Geometry: final body of the model. Coordinates: model frame, mm. Face numbers are marked on the shaded views. A direction names the side the tool comes from. Give positions to 0.01 mm unless a question says otherwise; leave off trailing zeros. One line per item, written item: value. Start each with the question number.
Autodesk Inventor part; units mm, degrees
ref_plane "YZ Plane" through (0, 0, 0) normal (1, 0, 0) x (0, 1, 0)
ref_plane "XZ Plane" through (0, 0, 0) normal (0, 1, 0) x (-1, 0, 0)
ref_plane "XY Plane" through (0, 0, 0) normal (0, 0, 1) x (1, 0, 0)
sketch "Sketch1" plane through (0, 0, 0) normal (0, 0, 1) x (1, 0, 0)
  line L0 (0, 0) -> (0, 190.5)
  line L1 (0, 190.5) -> (1.524, 190.5)
  line L2 (1.524, 190.5) -> (1.524, 260.35)
  line L3 (1.524, 260.35) -> (50.8, 260.35)
  line L4 (50.8, 260.35) -> (50.8, 187.325)
  line L5 (50.8, 187.325) -> (115.7676, 161.925)
  line L6 (115.7676, 161.925) -> (130.048, 161.925)
  line L7 (130.048, 161.925) -> (130.048, 0)
  line L8 (130.048, 0) -> (0, 0)
  line L9 (130.048, 160.3375) -> (0, 160.3375)
  dimension "d0" = 520.7
  dimension "d1" = 381
  dimension "d2" = 1.524
  dimension "d3" = 320.675
  dimension "d4" = 323.85
  dimension "d7" = 374.65
  dimension "d18" = 49.276
  dimension "d20" = 128.524
  dimension "d21" = 14.2804
revolve "Revolution1" add sketch "Sketch1" angle 360 about axis through (130.048, 0, 0) along (-1, 0, 0) contours L0 L1 L2 L3 L4 L5 L6 L7 L9
sketch "Sketch2" plane through (1.524, 0, 0) normal (-1, 0, 0) x (0, 0, 1)
  circle A0 centre (0, 0) radius 260.35
  circle A1 centre (0, 0) radius 190.5
  circle A2 centre (221.0935, 43.9782) radius 15.875
  line L0 (221.0935, 43.9782) -> (0, 0) construction
  circle A3 centre (0, 0) radius 225.425 construction
  line L1 (0, 0) -> (225.425, 0) construction
  dimension "d10" = 225.425
  dimension "d11" = 31.75
  dimension "d17" = 11.25
extrude "Extrusion1" cut sketch "Sketch2" against normal through all contours A2
pattern_circular "Circular Pattern1" count 16 over 360 about axis through (83.2838, 0, 0) along (1, 0, 0) of "Extrusion1"
chamfer "Chamfer1" distance 1.5875 angle 45 2 edges at (1.524, -260.35, 0) (50.8, -260.35, 0)
sketch "Sketch3" plane through (0, 0, 0) normal (0, 1, 0) x (-1, 0, 0)
  line L0 (-50.8, 187.325) -> (-115.7676, 161.925) construction
  line L1 (-115.7676, 161.925) -> (-130.048, 161.925) construction
  line L2 (-130.048, 160.3375) -> (0, 160.3375) construction
  line L3 (26.0096, 0) -> (-156.0576, 0)
  line L4 (-25.4, 160.3375) -> (-130.048, 160.3375)
  line L5 (-130.048, 160.3375) -> (-130.048, 165.1)
  line L6 (-130.048, 165.1) -> (-25.4, 165.1)
  line L7 (-25.4, 165.1) -> (-25.4, 160.3375)
  line L8 (-82.55, 165.1) -> (-82.55, 166.6875)
  line L9 (-82.55, 166.6875) -> (-74.0231, 177.8)
  line L10 (-74.0231, 177.8) -> (-71.4375, 177.8)
  arc A0 (-71.4375, 177.8) -> (-60.9321, 183.3637) centre (-71.4375, 190.5) ccw
  line L11 (-60.9321, 183.3637) -> (-130.048, 183.3637)
  line L12 (-130.048, 183.3637) -> (-130.048, 165.1)
  point P0 (0, 0)
  dimension "d25" = 25.4
  dimension "d26" = 330.2
  dimension "d27" = 355.6
  dimension "d28" = 1.5875
  dimension "d29" = 37.5
  dimension "d30" = 12.7
  dimension "d31" = 82.55
  dimension "d32" = 11.1125
  dimension "d33" = 2.5856
revolve "Revolution2" cut sketch "Sketch3" angle 360 about axis through (-10, 0, 0) along (1, 0, 0)
fillet "Fillet1" radius 0.7937 1 edges at (25.4, 0, -165.1)
chamfer "Chamfer2" distance 0.7937 angle 45 1 edges at (25.4, -160.3375, 0)
equation "\"d0\" = O"
equation "\"d1\" = R"
equation "\"d3\" = B"
equation "\"d4\" = A"
equation "\"d7\" = X"
equation "\"d18\" = C1"
equation "\"d20\" = Y"
equation "\"d21\" = 0.111111 * Y"
equation "\"d10\" = 0.5 * BC"
equation "\"d11\" = DH"
equation "\"O\" = 520.7"
equation "\"C1\" = 49.276"
equation "\"X\" = 374.65"
equation "\"A\" = 323.85"
equation "\"Y\" = 128.524"
equation "\"B\" = 320.675"
equation "\"BC\" = 450.85"
equation "\"DH\" = 31.75"
equation "\"R\" = 381"
properties part number "A1-19027-400-06 12in CL300 RFWN flange" material "Steel, Mild"
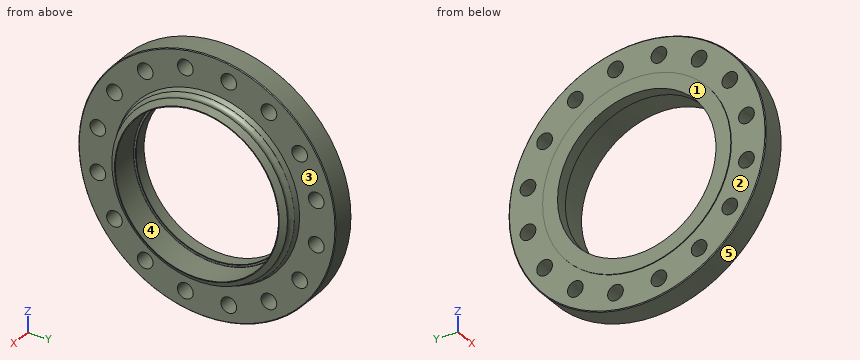
Item 1: Section A-A, the plane x = 13. State how many separate pieces and enclosed holes the cut face has, then the cut area to 3 significant figures.
Item 2: Access query for the marked faces 1 and 2. Directions: +Z, -Z, +X, -X, +Y, -Y. A direction counts if a zero-diameter tool reaches every point of the face in a straight line with its end or side. Return the directions, or none.
Item 3: Mould query, pull axis Z, two halves, no side actions, for the marked faces 3, 4 and 5. Classes: pulls with the +Z half, pulls with the -Z half, needs draft (parallel to the pull), parting line crosses it, or undercut.
Item 4: Pin query (flat end, axial travel): pin 1 (19 mm diameter, centred on y = 187.43, z = -125.24, fed in from +X); pin 2 (3 mm diameter, centred on x = 46.5, y = 61, fed in from +Z); pin 3 (4 mm diameter, centred on x = 53.5, z = -151.5, fed in from -Y); pin 4 (2 mm diameter, centred on x = 8.5, z = 178, fed in from -Y). Return the tip coordinate at first contact, or that it passes through.
Item 5: Ray query, line 1 along Z through (x, y) = (22, 119); line 2 along Y through (x, z) = (4, -49.5); line 3 along X through (y, z) = (-229, 19). Return the intervals inside material, ascending. Write a range as [from, to].
Geometry check:
1. separate pieces: 1
1. enclosed holes: 17
1. area: 120,000 mm2
2. face 1: +Z, -Z, -X, +Y, -Y
2. face 2: -X
3. face 3: needs draft
3. face 4: undercut
3. face 5: parting line crosses it
4. pin 1: passes through
4. pin 2: stops at z = 253.46
4. pin 3: stops at y = -111.41
4. pin 4: stops at y = -190.93
5. line 1: z = [-231.56, -202.03], [-172.84, -107.46], [107.46, 172.84], [202.03, 231.56]
5. line 2: y = [-255.6, -235.98], [-206.21, -152.51], [152.51, 206.21], [235.98, 255.6]
5. line 3: x = [1.52, 50.8]
